Source: CAD feature listing. Evaluate the final solid. Frame: model axes, mm. A direction names the side the tool comes from. Give positions to 0.01 mm unless a question says otherwise; leave off trailing zeros. Loops run counter-clockwise (first coordinate to the right, second up) from the corner with the lowest first, then second, coordinate; pieces in that order, holes last. Notation, with made-up numbers: (77, 1) -> (86, 1) arc R19 ccw to (86, 19) -> close; hole circle Ø3 at (74, -21). An arc over 180 degrees is marked (long way). Return JSON: item names as keys, results as strings. Group by question number.
(1) Cut plane C-C on y = 1.5. Return loops of the section in (x, z).
(2) Ray query, line 1 (Z direction, x = 4.75, y = 5); line 2 (Z direction, x = 4.25, y = 4.5); line 3 (Y direction, x = 17.25, z = -25). Return the intervals inside material, ascending. Write a range as from..to.
(3) Cut plane A-A on z = -25. Return loops of the section in (x, y), then the cut area to 3 significant figures.
(4) Cut plane B-B on x = 5. Return loops of the section in (y, z), then the cut area to 3 significant figures.
(5) Pin query (flat end, axial travel): pin 1 (1.5 mm diameter, centred on x = 3.5, z = -19.5, fed in from -Y). Return the tip coordinate at first contact, or that it passes through.
(6) Access query for faces 1 (the face through (10, 1, -22)), 2 (the face through (16.2, 5.1, -22.5)). Directions: +Z, -Z, +X, -X, +Y, -Y. A direction counts if a zero-diameter tool reaches every point of the face in a straight line with its end or side. Return the directions, or none.
(7) Draft query along Z for faces 3 (the face through (3.8, 8.614, -9.046)), 4 (the face through (10, 0, -43)), 5 (the face through (10, 5, -50)). Return one class per face: released by +Z, released by -Z, zero draft, split by the parting line, or undercut.
(8) Cut plane D-D on z = -10.5. Return loops of the section in (x, y), then the cut area to 3 significant figures.
```python
from build123d import *

# Parameters (mm, degrees)
ESQUISSE1_W             = 20
ESQUISSE1_H             = 50
ESQUISSE1_R             = 2.5
ESQUISSE1_R_2           = 1
BOSS_EXTRU_1_DEPTH      = 10
ESQUISSE2_R             = 2.5
ENL_V_MAT_EXTRU_1_DEPTH = 55.772255751
ENL_V_MAT_EXTRU_2_DEPTH = 41.175091243


with BuildPart() as part:
    # Esquisse1 → Boss.-Extru.1 (new body)
    with BuildSketch(Plane(origin=(0, 0, 0), x_dir=(1, 0, 0), z_dir=(0, 1, 0))):
        with Locations((10, 25)):
            Rectangle(ESQUISSE1_W, ESQUISSE1_H)
        with Locations(Location((10, 25, 0), (0, 0, 270))):
            Circle(ESQUISSE1_R, mode=Mode.SUBTRACT)
        with Locations(Location((11, 39, 0), (0, 0, 270))):
            Circle(ESQUISSE1_R, mode=Mode.SUBTRACT)
        with Locations(Location((9, 11, 0), (0, 0, 270))):
            Circle(ESQUISSE1_R, mode=Mode.SUBTRACT)
        with Locations(Location((16.5, 40, 0), (0, 0, 270))):
            Circle(ESQUISSE1_R_2, mode=Mode.SUBTRACT)
        with Locations(Location((3.5, 10, 0), (0, 0, 270))):
            Circle(ESQUISSE1_R_2, mode=Mode.SUBTRACT)
    extrude(amount=BOSS_EXTRU_1_DEPTH)

    # Esquisse2 → Enlèv. mat.-Extru.1 (cut, through all)
    with BuildSketch(Plane(origin=(20, 0, 0), x_dir=(0, 0, -1), z_dir=(1, 0, 0))):
        with Locations((11, 5)):
            Circle(ESQUISSE2_R)
        with Locations((25, 5)):
            Circle(ESQUISSE2_R)
        with Locations((39, 5)):
            Circle(ESQUISSE2_R)
    extrude(amount=-ENL_V_MAT_EXTRU_1_DEPTH, mode=Mode.SUBTRACT)

    # Esquisse3 → Enlèv. mat.-Extru.2 (cut, through all)
    with BuildSketch(Plane(origin=(0, -14.270103986, -25), x_dir=(0, 0, 1), z_dir=(-1, 0, 0))):
        with BuildLine():
            Line((-11.25, 14.270103986), (11.25, 14.270103986))
            Line((11.25, 14.270103986), (11.25, 14.770103986))
            ThreePointArc((11.25, 14.770103986), (11.103553391, 15.123657377), (10.75, 15.270103986))
            Line((10.75, 15.270103986), (-10.75, 15.270103986))
            ThreePointArc((-10.75, 15.270103986), (-11.103553391, 15.123657377), (-11.25, 14.770103986))
            Line((-11.25, 14.770103986), (-11.25, 14.270103986))
        make_face()
    extrude(amount=-ENL_V_MAT_EXTRU_2_DEPTH, mode=Mode.SUBTRACT)


solid = part.part
```
Answers:
{
 "1": {"outline": "(0, -50) -> (20, -50) -> (20, 0) -> (0, 0) -> close; hole circle Ø2 at (3.5, -10); hole circle Ø5 at (9, -11); hole circle Ø5 at (10, -25); hole circle Ø5 at (11, -39); hole circle Ø2 at (16.5, -40)"},
 "2": {"line 1": "-50..-41.5, -36.5..-27.5, -22.5..-13.5, -8.5..0", "line 2": "-50..-41.45, -36.55..-27.45, -22.55..-13.45, -8.55..0", "line 3": "1..2.5, 7.5..10"},
 "3": {"outline": "(0, 1) -> (7.5, 1) -> (7.5, 2.5) -> (0, 2.5) -> close; (0, 7.5) -> (7.5, 7.5) -> (7.5, 10) -> (0, 10) -> close; (12.5, 1) -> (20, 1) -> (20, 2.5) -> (12.5, 2.5) -> close; (12.5, 7.5) -> (20, 7.5) -> (20, 10) -> (12.5, 10) -> close", "area": "60.0 mm²"},
 "4": {"outline": "(0, -50) -> (10, -50) -> (10, 0) -> (0, 0) -> (0, -13.75) -> (0.5, -13.75) arc R0.5 cw to (1, -14.25) -> (1, -35.75) arc R0.5 cw to (0.5, -36.25) -> (0, -36.25) -> close; hole circle Ø5 at (5, -39); hole circle Ø5 at (5, -25); hole circle Ø5 at (5, -11)", "area": "419 mm²"},
 "5": {"pin 1": "y = 1"},
 "6": {"face 1": "+X, -X, -Y", "face 2": "+X, -X"},
 "7": {"face 3": "undercut", "face 4": "zero draft", "face 5": "released by -Z"},
 "8": {"outline": "(0, 0) -> (2.63, 0) -> (2.63, 2.55) -> (0, 2.55) -> close; (0, 7.45) -> (2.63, 7.45) -> (2.63, 10) -> (0, 10) -> close; (4.37, 0) -> (6.55, 0) -> (6.55, 2.55) -> (4.37, 2.55) -> close; (4.37, 7.45) -> (6.55, 7.45) -> (6.55, 10) -> (4.37, 10) -> close; (11.45, 0) -> (20, 0) -> (20, 2.55) -> (11.45, 2.55) -> close; (11.45, 7.45) -> (20, 7.45) -> (20, 10) -> (11.45, 10) -> close", "area": "68.2 mm²"}
}
